Could you check a few things on this drawing? It's one solid part, dimensions in mm from its lowest x, y, z. Round coordinates to 2 decimals unless told otherwise and drop trailing zeros. Write each loop counter-clockwise with the first axis right and the second up, starting at its lowest first coordinate (ties: lowest second). Pieces come first, ordered by that corner, then holes. Notation, with made-up numbers: (51, -27) -> (72, -27) arc R22 cw to (72, 9) -> close; hole circle Ø10 at (-6, 55). An arc over 180 degrees is marked (long way). Answer as CSV lines item,"result".
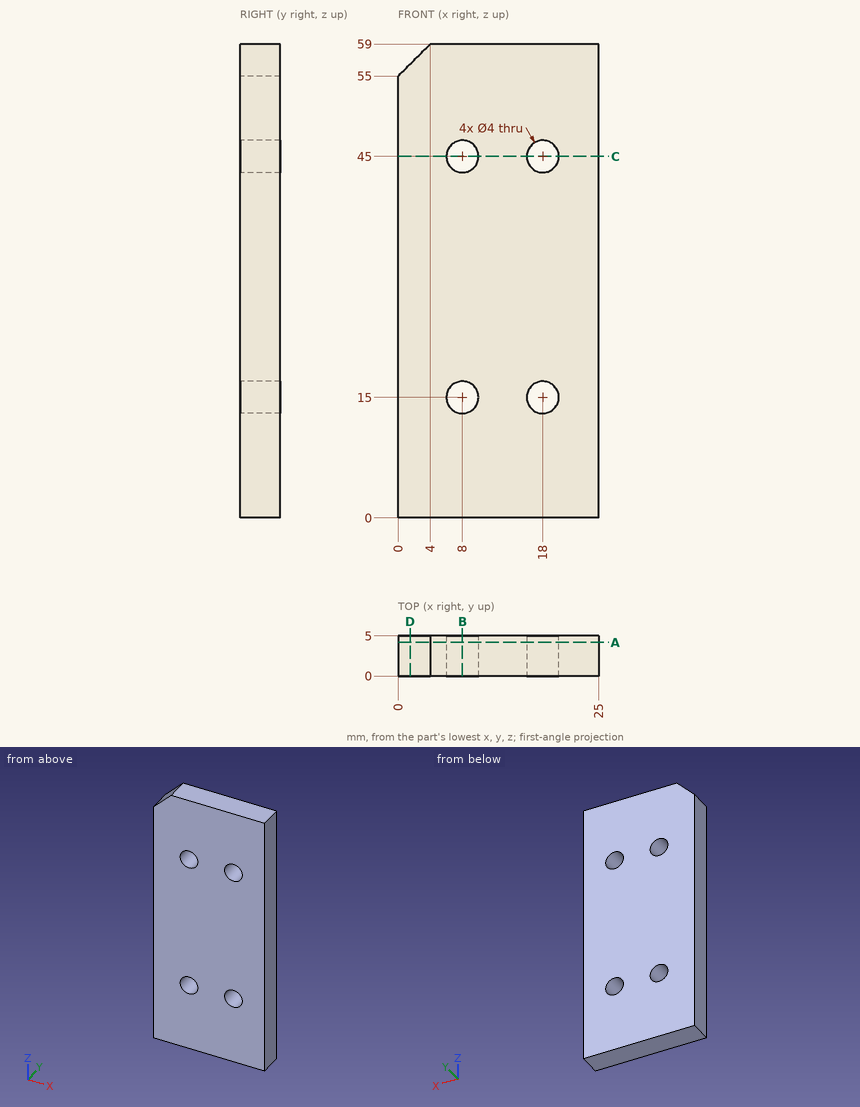
1. Suppose I cut it at A-A on y = 4.2. Please give me the cut outline in (x, z), and give its area (3 significant figures).
Numbers:
outline,"(0, 0) -> (25, 0) -> (25, 59) -> (4, 59) -> (0, 55) -> close; hole circle Ø4 at (8, 15); hole circle Ø4 at (8, 45); hole circle Ø4 at (18, 15); hole circle Ø4 at (18, 45)"
area,"1,420 mm^2"
2. Suppose I cut it at D-D on x = 1.5. Please give me the cut outline in (y, z).
Numbers:
outline,"(0, 0) -> (5, 0) -> (5, 56.5) -> (0, 56.5) -> close"
3. Suppose I cut it at C-C on z = 45. Please give me the cut outline in (x, y).
Numbers:
outline,"(0, 0) -> (6, 0) -> (6, 5) -> (0, 5) -> close; (10, 0) -> (16, 0) -> (16, 5) -> (10, 5) -> close; (20, 0) -> (25, 0) -> (25, 5) -> (20, 5) -> close"
4. If I drill on line 1 (Z direction, x = 18, y = 4); line 2 (Z direction, x = 16.75, y = 3.5); line 3 (X direction, y = 1.8, z = 16), over which ranges is the centre line in solid material (lowest first)?
Numbers:
line 1,"z = 0 to 13, 17 to 43, 47 to 59"
line 2,"z = 0 to 13.44, 16.56 to 43.44, 46.56 to 59"
line 3,"x = 0 to 6.27, 9.73 to 16.27, 19.73 to 25"
5. For pin 1 Ø3 at (x, y) = (10.5, 1) entering from -Z; pin 2 Ø2.5 at (x, z) = (18, 45) entering from -Y, each with a flat end and sliding along its axis, tell me the tip position at first contact or that it passes through.
Numbers:
pin 1,"stops at z = 0"
pin 2,"passes through"
6. Suppose I cut it at B-B on x = 8. Please give me the cut outline in (y, z), and give its area (3 significant figures).
Numbers:
outline,"(0, 0) -> (5, 0) -> (5, 13) -> (0, 13) -> close; (0, 17) -> (5, 17) -> (5, 43) -> (0, 43) -> close; (0, 47) -> (5, 47) -> (5, 59) -> (0, 59) -> close"
area,"255 mm^2"
